Model file for the job. Use its own axes, mm. Coordinates: 2 decimals unless noted, no trailing zeros. Write each loop counter-clockwise with the first axis right and the second up, starting at its lowest first coordinate (ties: lowest second). Pieces come first, ordered by that corner, then holes. Notation, with made-up numbers: M -35,33.5 L 13,33.5 A22 ccw 13,62.5 Z; hole C 65.25,42.5 d11. An arc over 180 degrees is marked long. Put each result on its own line as item: value. Start each with the question number.
Q1. Cut at C-C (y = 0). Write the cut outline in (x, z).
Q2. Drill centre lines: line 1 along Y through (x, z) = (25, 0.95); line 2 along X through (y, z) = (3.5, 0.5); line 3 along Y through (x, z) = (29.5, 0.1). Where is each one in solid material? Low to high.
Q3. Pull direction Y, two halves, no side cores. Call faces 1 (the flat face through (-40, 0, 1)), 2 (the flat face through (1, -14, 1)), 3 (the cylindrical face through (-14.5, -4.93, 0.79)): pulls with the +Y half, pulls with the -Y half, needs draft (parallel to the pull), parting line crosses it, or undercut.
Q4. Cut at A-A (x = -13). Write the cut outline in (y, z), then the cut area to 3 significant figures.
Q5. Drop a flat-ended pin along its axis: pin 1 (3.5 mm diameter, centred on x = -13, y = -5, fed in from -Z). Give the stop position or say it passes through.
Q6. Cut at D-D (x = 0). Write the cut outline in (y, z), then the cut area to 3 significant figures.
Q7. Cut at B-B (z = 0.25). Write the cut outline in (x, y), then the cut area to 3 significant figures.
```python
from build123d import *

# Parameters (mm, degrees)
SKETCH1_R           = 3
SKETCH1_R_2         = 6.5
SKETCH1_R_3         = 1.5
BOSS_EXTRUDE1_DEPTH = 1.6


with BuildPart() as part:
    # Sketch1 → Boss-Extrude1 (new body)
    with BuildSketch(Plane.XY):
        with BuildLine():
            Line((-36, 14), (36, 14))
            ThreePointArc((36, 14), (38.828427125, 12.828427125), (40, 10))
            Line((40, 10), (40, -10))
            ThreePointArc((40, -10), (38.828427125, -12.828427125), (36, -14))
            Line((36, -14), (-36, -14))
            ThreePointArc((-36, -14), (-38.828427125, -12.828427125), (-40, -10))
            Line((-40, -10), (-40, 10))
            ThreePointArc((-40, 10), (-38.828427125, 12.828427125), (-36, 14))
        make_face()
        with Locations((-26, 0)):
            Circle(SKETCH1_R, mode=Mode.SUBTRACT)
        Circle(SKETCH1_R_2, mode=Mode.SUBTRACT)
        with Locations((25, 0)):
            Circle(SKETCH1_R_2, mode=Mode.SUBTRACT)
        with Locations((-13, -5)):
            Circle(SKETCH1_R_3, mode=Mode.SUBTRACT)
    extrude(amount=BOSS_EXTRUDE1_DEPTH)


solid = part.part
```
Computed values:
1. outline: M -40,0 L -29,0 L -29,1.6 L -40,1.6 Z; M -23,0 L -6.5,0 L -6.5,1.6 L -23,1.6 Z; M 6.5,0 L 18.5,0 L 18.5,1.6 L 6.5,1.6 Z; M 31.5,0 L 40,0 L 40,1.6 L 31.5,1.6 Z
2. line 1: -14 to -6.5, 6.5 to 14
2. line 2: -40 to -5.48, 5.48 to 19.52, 30.48 to 40
2. line 3: -14 to -4.69, 4.69 to 14
3. face 1: needs draft
3. face 2: pulls with the -Y half
3. face 3: undercut
4. outline: M -14,0 L -6.5,0 L -6.5,1.6 L -14,1.6 Z; M -3.5,0 L 14,0 L 14,1.6 L -3.5,1.6 Z
4. area: 40.0 mm2
5. pin 1: z = 0
6. outline: M -14,0 L -6.5,0 L -6.5,1.6 L -14,1.6 Z; M 6.5,0 L 14,0 L 14,1.6 L 6.5,1.6 Z
6. area: 24.0 mm2
7. outline: M -40,-10 A4 ccw -36,-14 L 36,-14 A4 ccw 40,-10 L 40,10 A4 ccw 36,14 L -36,14 A4 ccw -40,10 Z; hole C -26,0 d6; hole C -13,-5 d3; hole C 0,0 d13; hole C 25,0 d13
7. area: 1,930 mm2
